from build123d import *

# Parameters (mm, degrees)
SKETCH_1_W          = 43.5
SKETCH_1_H          = 20.8
EXTRUDE_1_DEPTH     = 1.2
SKETCH_2_W          = 12
SKETCH_2_H          = 12
EXTRUDE_2_DEPTH     = 7.6
SKETCH_3_R          = 4
EXTRUDE_3_DEPTH     = 10.6
SKETCH_4_W          = 9.5
SKETCH_4_H          = 4.8
EXTRUDE_4_DEPTH     = 10
SKETCH_5_W          = 10.901177872
SKETCH_5_H          = 8.219839766
EXTRUDE_5_DEPTH     = 5
SKETCH_6_R          = 1.5
CUT_EXTRUDE_1_DEPTH = 5


with BuildPart() as part:
    # 草图1 → 凸台-拉伸1 (new body)
    with BuildSketch(Plane(origin=(0, 0, 0), x_dir=(1, 0, 0), z_dir=(0, 1, 0))):
        Rectangle(SKETCH_1_W, SKETCH_1_H)
    extrude(amount=EXTRUDE_1_DEPTH)

    # 草图2 → 凸台-拉伸2 (add)
    with BuildSketch(Plane(origin=(0, 1.2, 0), x_dir=(1, 0, 0), z_dir=(0, 1, 0))):
        with Locations((-5.75, 3.9)):
            Rectangle(SKETCH_2_W, SKETCH_2_H)
    extrude(amount=EXTRUDE_2_DEPTH)

    # 草图3 → 凸台-拉伸3 (add)
    with BuildSketch(Plane(origin=(0, 1.2, 0), x_dir=(1, 0, 0), z_dir=(0, 1, 0))):
        with Locations(Location((-17.25, 0, 0), (0, 0, 90))):
            Circle(SKETCH_3_R)
        with Locations(Location((17.25, 0, 0), (0, 0, 90))):
            Circle(SKETCH_3_R)
    extrude(amount=EXTRUDE_3_DEPTH)

    # 草图4 → 凸台-拉伸4 (add)
    with BuildSketch(Plane(origin=(0, 1.2, 0), x_dir=(1, 0, 0), z_dir=(0, 1, 0))):
        with Locations((-7, -7.5)):
            Rectangle(SKETCH_4_W, SKETCH_4_H)
    extrude(amount=EXTRUDE_4_DEPTH)

    # 草图5 → 凸台-拉伸5 (add)
    with BuildSketch(Plane(origin=(0, 1.2, 0), x_dir=(1, 0, 0), z_dir=(0, 1, 0))):
        with Locations((7.208843432, -2.703316287)):
            Rectangle(SKETCH_5_W, SKETCH_5_H)
    extrude(amount=EXTRUDE_5_DEPTH)

    # 草图6 → 切除-拉伸1 (cut)
    with BuildSketch(Plane(origin=(0, 1.2, 0), x_dir=(1, 0, 0), z_dir=(0, 1, 0))):
        with Locations(Location((15.25, -8.4, 0), (0, 0, 270))):
            Circle(SKETCH_6_R)
        with Locations(Location((-15.25, 8.4, 0), (0, 0, 270))):
            Circle(SKETCH_6_R)
    extrude(amount=-CUT_EXTRUDE_1_DEPTH, mode=Mode.SUBTRACT)


solid = part.part
The model under review builds one solid part; all positions refer to its coordinate system, in mm. A direction names the side the tool comes from. Give positions to 0.01 mm unless a question says otherwise; leave off trailing zeros. Loops run counter-clockwise (first coordinate to the right, second up) from the corner with the lowest first, then second, coordinate; pieces in that order, holes last. Notation, with made-up numbers: (40, 47.25) -> (95, 47.25) arc R18 cw to (95, 80.25) -> close; hole circle Ø9 at (50, 67.5). An arc over 180 degrees is marked (long way). Answer as a JSON object with one key per item and string values. Group by question number.
Q1. Take a section at A-A (y = 7.25). Write out the cut boundary in (x, z), plus the area to 3 significant figures.
Q2. Take a section at C-C (y = 4). Write out the cut boundary in (x, z), plus the area to 3 significant figures.
Q3. Wall thickness on line 1 along X through (y, z) = (0.75, -8.4); line 2 along Z through (x, y) = (-6.5, 1.75); line 3 along X through (y, z) = (0.45, 8.4): over which ranges is each line inside the solid? List them lowest first.
Q4. Take a section at B-B (z = 7.5). Write out the cut boundary in (x, y), plus the area to 3 significant figures.
Q5. Insertion check: pin 1 (5 mm diameter, centred on x = 6, y = 9.5, fed in from -Z); pin 2 (1.5 mm diameter, centred on x = 16, z = 7, fed in from +Y); pin 3 (6.5 mm diameter, centred on x = 6.5, z = 4, fed in from +Y); pin 4 (5 mm diameter, centred on x = -8.5, y = 8, fed in from -Z). Each pin has a flat end and moves straight along its axis. Give the tip position at first contact, or say it passes through.
Q6. Tool access review of faces 1 (the flat face through (-6, 5, -9.9)), 2 (the flat face through (7, 4, 6.813)), 3 (the flat face through (-6, 8.8, -4)): name each direction out of +Z, -Z, +X, -X, +Y, -Y from which nothing blocks a thin tool from reaching the whole face with its end or side.
Q7. Take a section at D-D (y = 10). Write out the cut boundary in (x, z), plus the area to 3 significant figures.
Q8. Draft analysis for pull direction Z (two halves, no side actions). For faces 4 (the flat face through (-6, 5, 2.1)), 5 (the flat face through (7, 4, -1.407)), 6 (the flat face through (-11.75, 6, 8)), state which applies: pulls with the +Z half, pulls with the -Z half, needs draft (parallel to the pull), parting line crosses it, or undercut.
Answer below:
{
 "1": {"outline": "circle Ø8 at (-17.25, 0); (-11.75, -9.9) -> (0.25, -9.9) -> (0.25, 2.1) -> (-11.75, 2.1) -> close; (-11.75, 5.1) -> (-2.25, 5.1) -> (-2.25, 9.9) -> (-11.75, 9.9) -> close; circle Ø8 at (17.25, 0)", "area": "290 mm2"},
 "2": {"outline": "circle Ø8 at (-17.25, 0); (-11.75, -9.9) -> (0.25, -9.9) -> (0.25, 2.1) -> (-11.75, 2.1) -> close; (-11.75, 5.1) -> (-2.25, 5.1) -> (-2.25, 9.9) -> (-11.75, 9.9) -> close; (1.76, -1.41) -> (12.66, -1.41) -> (12.66, 6.81) -> (1.76, 6.81) -> close; circle Ø8 at (17.25, 0)", "area": "380 mm2"},
 "3": {"line 1": "x = -21.75 to -16.75, -13.75 to 21.75", "line 2": "z = -9.9 to 2.1, 5.1 to 9.9", "line 3": "x = -21.75 to 13.75, 16.75 to 21.75"},
 "4": {"outline": "(-21.75, 0) -> (14.05, 0) -> (14.05, 1.2) -> (-2.25, 1.2) -> (-2.25, 11.2) -> (-11.75, 11.2) -> (-11.75, 1.2) -> (-21.75, 1.2) -> close; (16.45, 0) -> (21.75, 0) -> (21.75, 1.2) -> (16.45, 1.2) -> close", "area": "144 mm2"},
 "5": {"pin 1": "passes through", "pin 2": "stops at y = 1.2", "pin 3": "stops at y = 6.2", "pin 4": "stops at z = -9.9"},
 "6": {"face 1": "-Z, +X, -X, +Y", "face 2": "+Z, +X, +Y", "face 3": "-Z, +Y"},
 "7": {"outline": "circle Ø8 at (-17.25, 0); (-11.75, 5.1) -> (-2.25, 5.1) -> (-2.25, 9.9) -> (-11.75, 9.9) -> close; circle Ø8 at (17.25, 0)", "area": "146 mm2"},
 "8": {"face 4": "undercut", "face 5": "pulls with the -Z half", "face 6": "needs draft"}
}
